CAD build for the part. Positions are in the model's coordinates, mm. A direction names the side the tool comes from. Coordinates: 2 decimals unless noted, no trailing zeros. Write each loop counter-clockwise with the first axis right and the second up, starting at its lowest first coordinate (ties: lowest second). Pieces come first, ordered by that corner, then holes. Notation, with made-up numbers: (-17.5, 62) -> (7.5, 62) arc R19 cw to (7.5, 67) -> close; hole circle Ø7 at (-11.75, -14). An arc over 180 degrees is marked (long way). Answer as CSV lines item,"result".
```python
from build123d import *

# Parameters (mm, degrees)
F0_R     = 1.659583
F0_W     = 31.75
F0_H     = 1.27
F1_DEPTH = 50.8
F2_R     = 0.9525
F3_DEPTH = 38.1254
F5_DEPTH = 9.525


with BuildPart() as f1:
    # F0 (on Front) → F1 (new body, symmetric)
    with BuildSketch(Plane.XZ):
        Polygon((25.4, -9.525), (25.4, 8.255), (12.7, 8.255), (12.7, 6.985), (-25.4, 6.985), (-25.4, -9.525), align=None)
        with Locations((8.255, 4.199334)):
            Circle(F0_R, mode=Mode.SUBTRACT)
        Polygon((12.7, 8.255), (6.35, 8.255), (-25.4, 8.255), (-25.4, 6.985), (12.7, 6.985), align=None)
        with Locations((-9.525, 8.89)):
            Rectangle(F0_W, F0_H)
    extrude(amount=F1_DEPTH, both=True)

    # F2 (on face) → F3 (cut)
    with BuildSketch(Plane(origin=(-25.4, 0, 0), x_dir=(0, -1, 0), z_dir=(-1, 0, 0))):
        with Locations((0, 7.62)):
            Circle(F2_R)
    extrude(amount=-F3_DEPTH, mode=Mode.SUBTRACT)

    # F4 (on face) → F5 (cut)
    with BuildSketch(Plane.XY.offset(9.525)):
        with BuildLine():
            ThreePointArc((-13.97, 40.64), (-16.138026, 41.538026), (-15.24, 39.37))
            ThreePointArc((-15.24, 39.37), (-14.341974, 39.741974), (-13.97, 40.64))
        make_face()
        with BuildLine():
            ThreePointArc((-13.97, -40.64), (-14.341974, -39.741974), (-15.24, -39.37))
            ThreePointArc((-15.24, -39.37), (-16.138026, -41.538026), (-13.97, -40.64))
        make_face()
    extrude(amount=-F5_DEPTH, mode=Mode.SUBTRACT)


solid = f1.part
```
Item 1: Wall check: line 1 (Y direction, x = -15.24, z = 3); line 2 (X direction, y = 40.5, z = 0.75); line 3 (Z direction, x = 17.5, y = 31) (3 decimals). Give the ranges that are in metal, low to high. Write a range as from..to.
Answer below:
line 1,"y = -50.8..-41.91, -39.37..39.37, 41.91..50.8"
line 2,"x = -25.4..-16.5, -13.98..25.4"
line 3,"z = -9.525..8.255"
Item 2: Saw through at A-A on y = 21.5. Give the cut face in (x, z) (3 decimals), and give its area (3 significant figures).
Answer below:
outline,"(-25.4, -9.525) -> (25.4, -9.525) -> (25.4, 8.255) -> (6.35, 8.255) -> (6.35, 9.525) -> (-25.4, 9.525) -> close; hole circle Ø3.319 at (8.255, 4.199)"
area,"935 mm2"
Item 3: 3-axis set-ups, long thin cutter, end or side, ignore diameter. For faces 1 (the flat face through (-15, 41, 0)), 2 (the flat face through (16, -1, 8.255)), 3 (the flat face through (0, -50.8, 0)): which of +Z, -Z, +X, -X, +Y, -Y reach the whole face in a straight line?
Answer below:
face 1,"+Z"
face 2,"+Z, +X, +Y, -Y"
face 3,"+Z, -Z, +X, -X, -Y"
Item 4: Flat gauge pins, fed straight in: pin 1 (1 mm diameter, centred on y = 4, z = 9, fed in from +X); pin 2 (9.5 mm diameter, centred on x = 15, y = -14.5, fed in from +Z) (3 decimals). Where does each tip first touch, or does it go through?
Answer below:
pin 1,"stops at x = 6.35"
pin 2,"stops at z = 8.255"
Item 5: Two-plate mould, pull along Y, no slides. Class faces 4 (the flat face through (0, 50.8, 0)), 5 (the cylindrical face through (-6.6, 0.21, 6.69)), 6 (the flat face through (25.4, -1, -1)): pulls with the +Y half, pulls with the -Y half, needs draft (parallel to the pull), parting line crosses it, or undercut.
Answer below:
face 4,"pulls with the +Y half"
face 5,"undercut"
face 6,"needs draft"
